Geometry: final body of the model. Coordinates: model frame, mm. Face numbers are marked on the shaded views. Give positions to 0.01 mm unless a question says otherwise; leave off trailing zeros. Write each loop counter-clockwise with the first axis right and the second up, starting at its lowest first coordinate (ties: lowest second). Pieces come first, ordered by that corner, then holes.
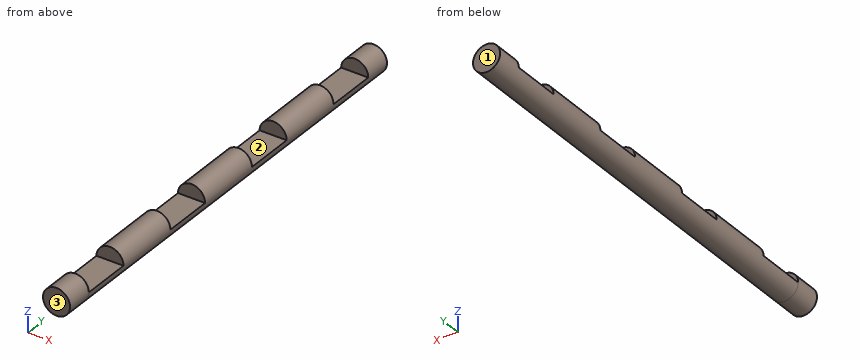
```python
from build123d import *

# Parameters (mm, degrees)
SKETCH1_R           = 13
BOSS_EXTRUDE1_DEPTH = 1
SKETCH16_R          = 13
BOSS_EXTRUDE3_DEPTH = 1
SKETCH19_R          = 1
BOSS_EXTRUDE4_DEPTH = 29.8
SKETCH18_W          = 22
SKETCH18_H          = 22
CUT_EXTRUDE6_DEPTH  = 3.7
SKETCH21_W          = 22
SKETCH21_H          = 22
CUT_EXTRUDE7_DEPTH  = 3.7
SKETCH22_W          = 22
SKETCH22_H          = 22
CUT_EXTRUDE8_DEPTH  = 3.7
SKETCH23_W          = 22
SKETCH23_H          = 22
CUT_EXTRUDE9_DEPTH  = 3.7
SKETCH24_R          = 19.921792127
CUT_EXTRUDE10_DEPTH = 1
SKETCH25_R          = 36.182885583
CUT_EXTRUDE11_DEPTH = 1
SKETCH26_R          = 1
BOSS_EXTRUDE5_DEPTH = 2
BOSS_EXTRUDE6_START = 2
SKETCH27_R          = 1
BOSS_EXTRUDE6_DEPTH = 2


with BuildPart() as part:
    # Sketch1 → Boss-Extrude1 (new body)
    with BuildSketch(Plane(origin=(0, 0, 0), x_dir=(1, 0, 0), z_dir=(0, 1, 0))):
        with Locations(Location((0, 0, 0), (0, 0, 270))):
            Circle(SKETCH1_R)
    extrude(amount=BOSS_EXTRUDE1_DEPTH)



with BuildPart() as body_2:
    # Sketch16 → Boss-Extrude3 (new body)
    with BuildSketch(Plane(origin=(0, 30.8, 0), x_dir=(1, 0, 0), z_dir=(0, 1, 0))):
        with Locations(Location((0, 0, 0), (0, 0, 270))):
            Circle(SKETCH16_R)
    extrude(amount=BOSS_EXTRUDE3_DEPTH)


with BuildPart() as part_1:
    add(part.part)

    add(body_2.part)  # Boss-Extrude4 merges body 2
    # Sketch19 → Boss-Extrude4 (add)
    with BuildSketch(Plane(origin=(0, 1, 0), x_dir=(1, 0, 0), z_dir=(0, 1, 0))):
        with Locations(Location((0, 11, 0), (0, 0, 270))):
            Circle(SKETCH19_R)
    extrude(amount=BOSS_EXTRUDE4_DEPTH)

    # Sketch18 → Cut-Extrude6 (cut)
    with BuildSketch(Plane(origin=(0, 4.7, 0), x_dir=(1, 0, 0), z_dir=(0, 1, 0))):
        Rectangle(SKETCH18_W, SKETCH18_H)
    extrude(amount=-CUT_EXTRUDE6_DEPTH, mode=Mode.SUBTRACT)

    # Sketch21 → Cut-Extrude7 (cut)
    with BuildSketch(Plane(origin=(0, 13.4, 0), x_dir=(1, 0, 0), z_dir=(0, 1, 0))):
        Rectangle(SKETCH21_W, SKETCH21_H)
    extrude(amount=-CUT_EXTRUDE7_DEPTH, mode=Mode.SUBTRACT)

    # Sketch22 → Cut-Extrude8 (cut)
    with BuildSketch(Plane(origin=(0, 22.1, 0), x_dir=(1, 0, 0), z_dir=(0, 1, 0))):
        Rectangle(SKETCH22_W, SKETCH22_H)
    extrude(amount=-CUT_EXTRUDE8_DEPTH, mode=Mode.SUBTRACT)

    # Sketch23 → Cut-Extrude9 (cut)
    with BuildSketch(Plane(origin=(0, 30.8, 0), x_dir=(1, 0, 0), z_dir=(0, 1, 0))):
        Rectangle(SKETCH23_W, SKETCH23_H)
    extrude(amount=-CUT_EXTRUDE9_DEPTH, mode=Mode.SUBTRACT)

    # Sketch24 → Cut-Extrude10 (cut)
    with BuildSketch(Plane(origin=(0, 31.8, 0), x_dir=(1, 0, 0), z_dir=(0, 1, 0))):
        Circle(SKETCH24_R)
    extrude(amount=-CUT_EXTRUDE10_DEPTH, mode=Mode.SUBTRACT)

    # Sketch25 → Cut-Extrude11 (cut)
    with BuildSketch(Plane(origin=(0, 1, 0), x_dir=(1, 0, 0), z_dir=(0, 1, 0))):
        Circle(SKETCH25_R)
    extrude(amount=-CUT_EXTRUDE11_DEPTH, mode=Mode.SUBTRACT)

    # Sketch26 → Boss-Extrude5 (add)
    with BuildSketch(Plane(origin=(0, 30.8, 0), x_dir=(1, 0, 0), z_dir=(0, 1, 0))):
        with Locations((0, 11)):
            Circle(SKETCH26_R)
    extrude(amount=BOSS_EXTRUDE5_DEPTH)

    # Sketch27 → Boss-Extrude6 (add)
    with BuildSketch(Plane.XZ.offset(-1).offset(BOSS_EXTRUDE6_START)):
        with Locations(Location((0, -11, 0), (0, 0, 270))):
            Circle(SKETCH27_R)
    extrude(amount=-BOSS_EXTRUDE6_DEPTH)


solid = part_1.part
```
Item 1: Section B-B, the plane y = 3. Return the cut outline in (x, z), plus the area to 3 significant figures.
Found:
outline: (-1, -11) arc R1 ccw to (1, -11) - close
area: 1.57 mm2
Item 2: Pull-direction query (Y, two-part tool) for the marked faces 1, 2 and 3; classes: +Y half, -Y half, draft (parallel to the pull), parting line (faces both ways), or undercut.
Found:
face 1: +Y half
face 2: undercut
face 3: -Y half
Item 3: Line query: L1, parallel to Y at x = -0.6, z = -10.9; L2, parallel to X at y = 19, z = -11.05; L3, parallel to X at y = 9.5, z = -11.5. Output: solid intervals per line, ascending.
Found:
L1: y = -1 to 1, 4.7 to 9.7, 13.4 to 18.4, 22.1 to 27.1, 30.8 to 32.8
L2: x = -1 to 1
L3: x = -0.87 to 0.87
Item 4: Section C-C, the plane y = 7. Return the cut outline in (x, z), plus the area to 3 significant figures.
Found:
outline: circle Ø2 at (0, -11)
area: 3.14 mm2
Item 5: Pin query (flat end, axial travel): pin 1 Ø0.6 at (x, y) = (0, 3) entering from +Z; pin 2 Ø1 at (x, y) = (-0.5, 8.5) entering from +Z; pin 3 Ø1 at (x, y) = (-1, 11) entering from -Z. Return the tip coordinate at first contact, or that it passes through.
Found:
pin 1: stops at z = -11
pin 2: stops at z = -10
pin 3: stops at z = -11.87
